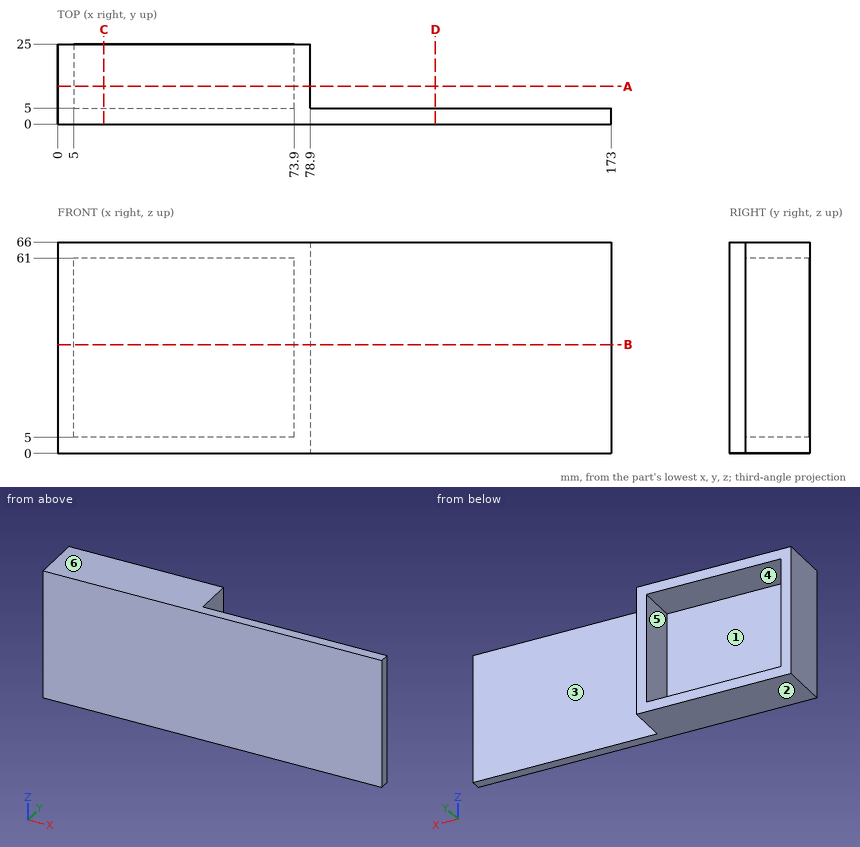
Verification items for this drawing (mm, ordinates from the low corner). A direction names the side the tool comes from. Round coordinates to 2 decimals unless told otherwise and drop trailing zeros. Loops run counter-clockwise (first coordinate to the right, second up) from the corner with the lowest first, then second, coordinate; pieces in that order, holes last. Notation, with made-up numbers: M 69.5,16 L 95.5,16 A18 cw 95.5,37 Z; hole C -9,-13.75 d6. An arc over 180 degrees is marked long. Answer as a JSON object with one key per item and string values.
1. Section check A-A (y = 11.75). Record the boundary of the cut face in (x, z), plus the area to 3 significant figures.
Reply:
{"outline": "M 0,0 L 78.9,0 L 78.9,66 L 0,66 Z; hole M 5,5 L 73.9,5 L 73.9,61 L 5,61 Z", "area": "1,350 mm²"}
2. Section check C-C (x = 14.5). Record the boundary of the cut face in (y, z).
Reply:
{"outline": "M 0,0 L 25,0 L 25,5 L 5,5 L 5,61 L 25,61 L 25,66 L 0,66 Z"}
3. Section check B-B (z = 34). Record the boundary of the cut face in (x, y), plus the area to 4 significant figures.
Reply:
{"outline": "M 0,0 L 173,0 L 173,5 L 78.9,5 L 78.9,25 L 73.9,25 L 73.9,5 L 5,5 L 5,25 L 0,25 Z", "area": "1,065 mm²"}
4. Mould release check, pull along Z, two halves, no side actions. Record for the marked faces 3, 4, 5 and 6: pulls with the +Z half, pulls with the -Z half, needs draft (parallel to the pull), parting line crosses it, or undercut.
Reply:
{"face 3": "needs draft", "face 4": "undercut", "face 5": "undercut", "face 6": "pulls with the +Z half"}
5. Gauge pin test, flat ends, axial feed: P1, Ø10, axis at x = 60, z = 39, coming from the -Y side; P2, Ø4, axis at x = 42, z = 28, coming from the +Y side; P3, Ø6, axis at y = 17.5, z = 40.5, coming from the +X side. Record the tip position at first contact, or that the pin passes through.
Reply:
{"P1": "stops at y = 0", "P2": "stops at y = 5", "P3": "stops at x = 78.9"}
6. Scan lines: line 1 (Z direction, x = 37.5, y = 17.25); line 2 (X direction, y = 12.5, z = 36); line 3 (Y direction, x = 37, z = 56). Record each from-to range of solid material in increasing order.
Reply:
{"line 1": "z = 0 to 5, 61 to 66", "line 2": "x = 0 to 5, 73.9 to 78.9", "line 3": "y = 0 to 5"}
7. Access from +Z, -Z, +X, -X, +Y, -Y to the whole of each face (thin tool, end or side, straight path). Record for the marked faces 1 and 2.
Reply:
{"face 1": "+Y", "face 2": "-Z, +X, -X, +Y, -Y"}
8. Section check D-D (x = 118). Record the boundary of the cut face in (y, z).
Reply:
{"outline": "M 0,0 L 5,0 L 5,66 L 0,66 Z"}
